Autodesk Inventor part; units mm, degrees
ref_plane "YZ Plane" through (0, 0, 0) normal (1, 0, 0) x (0, 1, 0)
ref_plane "XZ Plane" through (0, 0, 0) normal (0, 1, 0) x (-1, 0, 0)
ref_plane "XY Plane" through (0, 0, 0) normal (0, 0, 1) x (1, 0, 0)
sketch "Sketch1" plane through (0, 0, 0) normal (0, 1, 0) x (-1, 0, 0)
  line L0 (-90, 90) -> (90, 90)
  line L1 (90, 90) -> (90, -90)
  line L2 (90, -90) -> (-90, -90)
  line L3 (-90, -90) -> (-90, 90)
  line L4 (45.0987, -90) -> (90, -45.0987)
  line L5 (45.0987, -90) -> (108.5987, -90) construction
  point P0 (0, 0)
  point P1 (-90.1, 76.6)
  dimension "d3" = 90
  dimension "d4" = 90
  dimension "d5" = 90
  dimension "d6" = 90
  dimension "d7" = 45
  dimension "d8" = 31.75
  dimension "d9" = 180
extrude "Extrusion1" add sketch "Sketch1" along normal blind 2.5 contours L0 L1 L4 L2 L3
properties part number "Lid_Clear_Model"
The model under review builds one solid part; all positions refer to its coordinate system, in mm. Round coordinates to 2 decimals unless told otherwise and drop trailing zeros. Write each loop counter-clockwise with the first axis right and the second up, starting at its lowest first coordinate (ties: lowest second). Pieces come first, ordered by that corner, then holes. Notation, with made-up numbers: M 78.5,-15 L 84.5,-15 A23 cw 84.5,17 Z; hole C 32.5,27.25 d9. An arc over 180 degrees is marked long. Use CSV: the item, a comma, the result in double quotes. Start each with the question number.
(1) Clearance check with a flat-ended pin moving along its axis: P1, Ø1.5, axis at x = -7, z = -45.5, coming from the -Y side. State where the tip first meets the part, or that it passes through.
(2) We need section A-A, the plane y = 1.7. State the section outline as (x, z) points, then the cut area to 3 significant figures.
(3) We need section C-C, the plane x = -60.5. State the section outline as (y, z) points, then the cut area to 3 significant figures.
(4) We need section B-B, the plane z = -77. State the section outline as (x, y) points, then the cut area to 3 significant figures.
(5) For line 1 along X through (y, z) = (1.75, -70); line 2 along Z through (x, y) = (-54, 1); line 3 along Z through (x, y) = (-66.5, 1.6), list the stretches that pass through material, from the lowest coordinate up.
Findings:
1,P1,"y = 0"
2,outline,"M -90,-45.1 L -45.1,-90 L 90,-90 L 90,90 L -90,90 Z"
2,area,"31,400 mm^2"
3,outline,"M 0,-74.6 L 2.5,-74.6 L 2.5,90 L 0,90 Z"
3,area,"411 mm^2"
4,outline,"M -58.1,0 L 90,0 L 90,2.5 L -58.1,2.5 Z"
4,area,"370 mm^2"
5,line 1,"-65.1 to 90"
5,line 2,"-81.1 to 90"
5,line 3,"-68.6 to 90"
